CAD build for the part. Positions are in the model's coordinates, mm. Face numbers are marked on the shaded views. A direction names the side the tool comes from. Coordinates: 2 decimals unless noted, no trailing zeros. Loops run counter-clockwise (first coordinate to the right, second up) from the corner with the lowest first, then second, coordinate; pieces in that order, holes last. Notation, with made-up numbers: (54, -3.5) - (106, -3.5) arc R20 cw to (106, 26.5) - close; hole circle Ø8 at (52, -8.5). An arc over 180 degrees is marked (long way). Put each result on its own line as item: value.
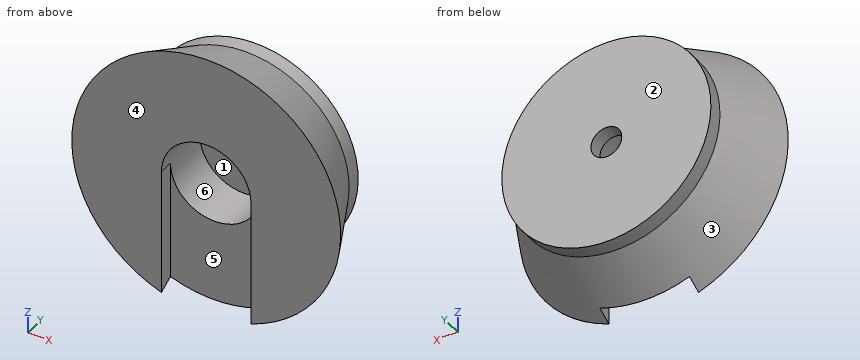
```python
from build123d import *

# Parameters (mm, degrees)
CROQUIS3_R              = 35
SALIENTE_EXTRUIR1_DEPTH = 5
CROQUIS4_R              = 5.16
CORTAR_EXTRUIR1_DEPTH   = 69.806581081
CROQUIS5_R              = 15
CORTAR_EXTRUIR2_DEPTH   = 21.16
CORTAR_EXTRUIR4_DEPTH   = 5


with BuildPart() as part:
    # Croquis2 → Revolución1 (revolve)
    with BuildSketch(Plane.XY, mode=Mode.PRIVATE) as revoluci_n1_sk:
        Polygon((0, -38.041888008), (-45, -38.041888008), (-35, -16.881888008), (0, -16.881888008), align=None)
    revolve(revoluci_n1_sk.sketch.rotate(Axis((0, 0, 0), (0, -1, 0)), 270), axis=Axis((0, 0, 0), (0, -1, 0)))

    # Croquis3 → Saliente-Extruir1 (add)
    with BuildSketch(Plane(origin=(0, -16.881888008, 0), x_dir=(1, 0, 0), z_dir=(0, 1, 0))):
        with Locations(Location((0, 0, 0), (0, 0, 270))):
            Circle(CROQUIS3_R)
    extrude(amount=SALIENTE_EXTRUIR1_DEPTH)

    # Croquis4 → Cortar-Extruir1 (cut, through all)
    with BuildSketch(Plane(origin=(0, -11.881888008, 0), x_dir=(1, 0, 0), z_dir=(0, 1, 0))):
        with Locations(Location((0, 0, 0), (0, 0, 270))):
            Circle(CROQUIS4_R)
    extrude(amount=-CORTAR_EXTRUIR1_DEPTH, mode=Mode.SUBTRACT)

    # Croquis5 → Cortar-Extruir2 (cut)
    with BuildSketch(Plane.XZ.offset(38.041888008)):
        with Locations(Location((0, 0, 0), (0, 0, 270))):
            Circle(CROQUIS5_R)
    extrude(amount=-CORTAR_EXTRUIR2_DEPTH, mode=Mode.SUBTRACT)

    # Croquis6 → Cortar-Extruir4 (cut)
    with BuildSketch(Plane.XZ.offset(38.041888008)):
        with BuildLine():
            Line((15, 0), (-15, 0))
            Line((-15, 0), (-15, -42.426406871))
            add(Edge.make_bspline(
                [(-15, -42.426406871), (-10.19808837, -44.127599643), (-0.005080405, -45.873007121), (10.203817441, -44.12638642), (15, -42.426406871)],
                knots=[0, 0, 0, 0, 0.500054305, 1, 1, 1, 1], degree=3))
            Line((15, -42.426406871), (15, 0))
        make_face()
    extrude(amount=-CORTAR_EXTRUIR4_DEPTH, mode=Mode.SUBTRACT)


with BuildPart() as cortar_extruir4_kept_piece:
    # of the separate pieces the step leaves, the one the design keeps (cortar_extruir4_pieces_kept)
    add(part.part.solids().sort_by_distance((0, -38.041888008, 45))[0])


solid = cortar_extruir4_kept_piece.part
```
Q1. Mould opens along X. For the marked faces 1, 2 and 3 say: +X half, -X half, draft (parallel to the pull), parting line (faces both ways), or undercut.
Determined:
face 1: undercut
face 2: draft
face 3: parting line
Q2. Slice it at A-A, the plane x = 0. Give the cut face in (y, z), then the cut area to 3 significant figures.
Determined:
outline: (-38.04, 15) - (-16.88, 15) - (-16.88, 5.16) - (-11.88, 5.16) - (-11.88, 35) - (-16.88, 35) - (-38.04, 45) - close; (-33.04, -42.64) - (-16.88, -35) - (-11.88, -35) - (-11.88, -5.16) - (-16.88, -5.16) - (-16.88, -15) - (-33.04, -15) - close
area: 1,210 mm2
Q3. Wall check: L1, parallel to X at y = -15.05, z = 0; L2, parallel to Z at x = 10, y = -22.25; L3, parallel to Z at x = 1, y = -18. Give the ranges that are in metal, low to high. Write a range as from..to.
Determined:
L1: -35..-5.16, 5.16..35
L2: -36.18..-11.18, 11.18..36.18
L3: -35.51..-14.97, 14.97..35.51
Q4. Pin check, flat tips, straight feed: pin 1 Ø1.5 at (y, z) = (-36.5, -21.5) entering from +X; pin 2 Ø10 at (x, z) = (10.5, -28.5) entering from -Y; pin 3 Ø6 at (y, z) = (-14.5, 14.5) entering from -X; pin 4 Ø2.5 at (y, z) = (-35.5, -20.5) entering from -X. Stop position of each tip, or through.
Determined:
pin 1: x = 39.27
pin 2: y = -38.04
pin 3: x = -33.06
pin 4: x = -39.63
Q5. Slice it at B-B, the plane y = -31.75. Give the cut face in (x, z).
Determined:
outline: circle Ø84.05 at (0, 0); hole circle Ø30 at (0, 0)
Q6. Slice it at C-C, the plane y = -15.5. Give the cut face in (x, z).
Determined:
outline: circle Ø70 at (0, 0); hole circle Ø10.32 at (0, 0)
Q7. Tool access for the marked faces 4, 5 and 6: list every direction of +Z, -Z, +X, -X, +Y, -Y with a clear straight run to the whole face (end or side of a thin tool).
Determined:
face 4: +Z, -Z, +X, -X, -Y
face 5: -Z, -Y
face 6: -Y
